Here's the drawing with two shaded views (mm, measured from the low corner). I have some questions. A direction names the side the tool comes from. Give positions to 0.01 mm unless a question says otherwise; leave off trailing zeros. Loops run counter-clockwise (first coordinate to the right, second up) from the corner with the lowest first, then second, coordinate; pieces in that order, holes last. Notation, with made-up numbers: (19, -9) - (48, -9) arc R14 cw to (48, 4) - close; hole circle Ø11 at (15.5, 68). An arc over 180 degrees is marked (long way). Use one line per item in the form item = value.
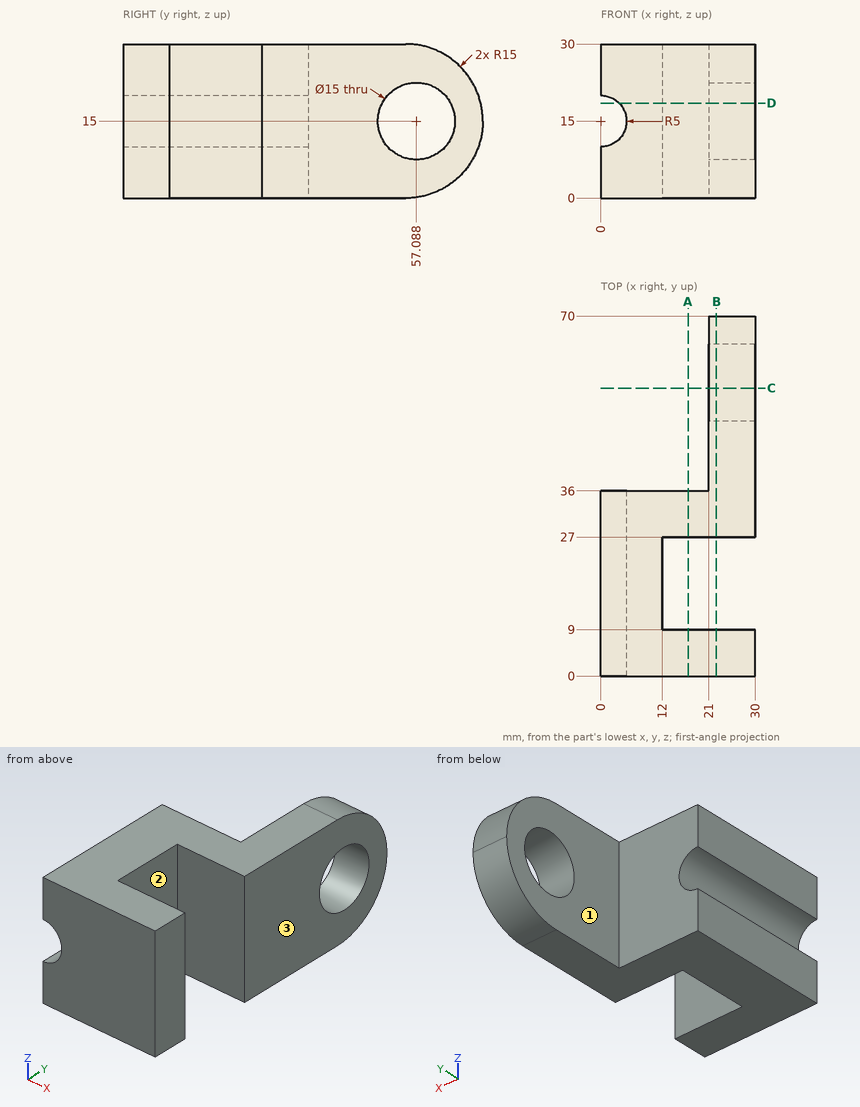
(1) If I drill on probe 1 along Y at (x, z) = (28.25, 15); probe 2 along Y at (x, z) = (15.5, 7.5); probe 3 along Y at (x, z) = (24.5, 17.5), over which ranges is the centre line in solid material (lowest first)?
Geometry says:
probe_1 = 0 to 9, 27 to 49.59, 64.59 to 70
probe_2 = 0 to 9, 27 to 36
probe_3 = 0 to 9, 27 to 50.02, 64.16 to 69.79
(2) For P1, Ø17, axis at x = 11.5, z = 9, coming from the +Y side; P2, Ø12, axis at y = 57.09, z = 15, coming from the -X side; P3, Ø5.5, axis at y = 18, z = 16.5, coming from the +X side; P4, Ø9, axis at y = 48, z = 15, coming from the -X side, each with a flat end and sliding along its axis, tell me the tip position at first contact or that it passes through.
Geometry says:
P1 = 36
P2 = through
P3 = 12
P4 = 21
(3) If we section it at C-C (y = 56): List the corners of the cut face in (x, z) for me.
Geometry says:
outline = (21, 0.03) - (30, 0.03) - (30, 7.58) - (21, 7.58) - close; (21, 22.42) - (30, 22.42) - (30, 29.97) - (21, 29.97) - close
(4) If we section it at A-A (x = 17): List the corners of the cut face in (y, z) for me.
Geometry says:
outline = (0, 0) - (9, 0) - (9, 30) - (0, 30) - close; (27, 0) - (36, 0) - (36, 30) - (27, 30) - close
(5) If we section it at B-B (x = 22.5): Give the number of separate pieces and of enclosed holes in the cut face, plus the area to 3 significant figures.
Geometry says:
separate_pieces = 2
enclosed_holes = 1
area = 1,290 mm²
(6) If we section it at D-D (z = 18.5): List the corners of the cut face in (x, y) for me, plus the area to 3 significant figures.
Geometry says:
outline = (3.57, 0) - (30, 0) - (30, 9) - (12, 9) - (12, 27) - (30, 27) - (30, 50.45) - (21, 50.45) - (21, 36) - (3.57, 36) - close; (21, 63.72) - (30, 63.72) - (30, 69.59) - (21, 69.59) - close
area = 810 mm²
(7) For the marked faces 1, 2 and 3, which set-ups out of +Z, -Z, +X, -X, +Y, -Y let a thin tool reach every point of the face, with its end or its side?
Geometry says:
face_1 = +Z, -Z, -X, +Y
face_2 = +Z, -Z, +X
face_3 = +Z, -Z, +X, +Y, -Y
